```python
from build123d import *

# Parameters (mm, degrees)
SKETCH_1_W          = 71.15
SKETCH_1_H          = 94.15
EXTRUDE_1_DEPTH     = 0.55
SKETCH_2_W          = 0.55
SKETCH_2_H          = 94.15
EXTRUDE_2_DEPTH     = 9.5
SKETCH_3_W          = 10
SKETCH_3_H          = 9.6
EXTRUDE_3_DEPTH     = 0.55
SKETCH_4_R          = 1.45
CUT_EXTRUDE_1_DEPTH = 0.55
EXTRUDE_4_DEPTH     = 71.15
SKETCH_6_W          = 5.65
SKETCH_6_H          = 0.55
EXTRUDE_5_DEPTH     = 2.3


with BuildPart() as part:
    # Эскиз1 → Бобышка-Вытянуть1 (new body)
    with BuildSketch(Plane(origin=(0, 0, 0), x_dir=(1, 0, 0), z_dir=(0, 1, 0))):
        Rectangle(SKETCH_1_W, SKETCH_1_H)
    extrude(amount=EXTRUDE_1_DEPTH)

    # Эскиз2 → Бобышка-Вытянуть2 (add)
    with BuildSketch(Plane.XZ):
        with Locations((-35.3, 0)):
            Rectangle(SKETCH_2_W, SKETCH_2_H)
        with Locations((35.3, 0)):
            Rectangle(SKETCH_2_W, SKETCH_2_H)
    extrude(amount=EXTRUDE_2_DEPTH)

    # Эскиз3 → Бобышка-Вытянуть3 (add)
    with BuildSketch(Plane(origin=(0, 0.55, 0), x_dir=(1, 0, 0), z_dir=(0, 1, 0))):
        with Locations((-28.625, 51.875)):
            Rectangle(SKETCH_3_W, SKETCH_3_H)
    extrude(amount=-EXTRUDE_3_DEPTH)

    # Эскиз4 → Вырез-Вытянуть1 (cut)
    with BuildSketch(Plane(origin=(0, 0.55, 0), x_dir=(1, 0, 0), z_dir=(0, 1, 0))):
        with Locations(Location((-28.575, 51.625, 0), (0, 0, 270))):
            Circle(SKETCH_4_R)
    extrude(amount=-CUT_EXTRUDE_1_DEPTH, mode=Mode.SUBTRACT)

    # Эскиз5 → Бобышка-Вытянуть4 (add)
    with BuildSketch(Plane.ZY.offset(35.575)):
        Polygon((42.075, 0.55), (42.075, 1.1), (53.125, 1.1), (53.125, -9.5), (52.575, -9.5), (52.575, 0.55), align=None)
    extrude(amount=-EXTRUDE_4_DEPTH)

    # Эскиз6 → Бобышка-Вытянуть5 (add)
    with BuildSketch(Plane.ZY.offset(35.575)):
        with Locations((-21.9, -5.975)):
            Rectangle(SKETCH_6_W, SKETCH_6_H)
        with Locations((32.7, -5.975)):
            Rectangle(SKETCH_6_W, SKETCH_6_H)
    extrude_5 = extrude(amount=EXTRUDE_5_DEPTH)

    # Зеркальное отражение1: Бобышка-Вытянуть5 across plane
    add(extrude_5.mirror(Plane(origin=(0, 0, 0), x_dir=(0, 0, 1), z_dir=(1, 0, 0))))


solid = part.part
```
Geometry: final body of the model. Coordinates: model frame, mm. A direction names the side the tool comes from. Coordinates: 2 decimals unless noted, no trailing zeros. Order: outer loops, then holes, each group sorted by start corner. A loop starts at its lowest first (then second) coordinate and runs counter-clockwise, first axis right, second up. Notation, with made-up numbers: M -18,47.25 L -11,47.25 A20 ccw -11,79.25 Z; hole C 60.5,-13.75 d1. An arc over 180 degrees is marked long. Answer as CSV lines item,"result".
Q1. Section B-B on z = -26. Return the cut outline in (x, y) (3 decimals).
Answers:
outline,"M -35.575,-9.5 L -35.025,-9.5 L -35.025,0 L 35.025,0 L 35.025,-9.5 L 35.575,-9.5 L 35.575,0.55 L -35.575,0.55 Z"
Q2. Section D-D on x = -16. Return the cut outline in (y, z) (3 decimals).
Answers:
outline,"M -9.5,52.575 L 0.55,52.575 L 0.55,47.075 L 0,47.075 L 0,-47.075 L 0.55,-47.075 L 0.55,42.075 L 1.1,42.075 L 1.1,53.125 L -9.5,53.125 Z"
Q3. Line query: probe 1 along X at (y, z) = (-7, -0.5) (3 decimals); probe 2 along Z at (x, y) = (-21.5, 0.5) (3 decimals); probe 3 along Y at (x, z) = (18, -10.5). Output: solid intervals per line, ascending. Write a range as [from, to].
Answers:
probe 1,"x = [-35.575, -35.025], [35.025, 35.575]"
probe 2,"z = [-47.075, 47.075], [52.575, 53.125]"
probe 3,"y = [0, 0.55]"
Q4. Draft query along X for faces 1 (the flat face through (0, 0, -6)), 2 (the flat face through (-37, -5.7, 33)). Return one class per face: pulls with the +X half, pulls with the -X half, needs draft (parallel to the pull), parting line crosses it, or undercut.
Answers:
face 1,"undercut"
face 2,"needs draft"
Q5. Section C-C on x = -26. Return the cut outline in (y, z) (3 decimals), and give its area (3 significant figures).
Answers:
outline,"M -9.5,52.575 L 0.55,52.575 L 0.55,47.075 L 0,47.075 L 0,-56.675 L 0.55,-56.675 L 0.55,42.075 L 1.1,42.075 L 1.1,53.125 L -9.5,53.125 Z"
area,"68.7 mm^2"
Q6. First-contact query: P1, Ø1, axis at x = -17.5, y = -2, coming from the -Z side (3 decimals); P2, Ø3, axis at y = -5, z = 14, coming from the +X side (3 decimals); P3, Ø1.8, axis at x = 37, z = 32, coming from the -Y side; P4, Ø2.5, axis at x = -36.5, z = 32.5, coming from the -Y side. Flat tips, straight axial feed; report the tip coordinate or a pass-through.
Answers:
P1,"stops at z = 52.575"
P2,"stops at x = 35.575"
P3,"stops at y = -6.25"
P4,"stops at y = -9.5"
Q7. Set-up query: faces 3 (the flat face through (37, -5.7, 33)), 4 (the flat face through (0, 0.55, 50)), 5 (the flat face through (0, 0.55, -8)), 6 (the flat face through (35.025, -5, -1)), 7 (the flat face through (-37, -5.7, -22)). Return all of +Z, -Z, +X, -X, +Y, -Y with unobstructed straight access to the full face (end or side cutting, diameter ignored); none if empty.
Answers:
face 3,"+Z, -Z, +X, +Y"
face 4,"+X, -X, -Y"
face 5,"-Z, +X, -X, +Y"
face 6,"-Z, -Y"
face 7,"+Z, -Z, -X, +Y"
Q8. Section A-A on y = -3.75. Return the cut outline in (x, z) (3 decimals).
Answers:
outline,"M -35.575,-47.075 L -35.025,-47.075 L -35.025,47.075 L -35.575,47.075 Z; M -35.575,52.575 L 35.575,52.575 L 35.575,53.125 L -35.575,53.125 Z; M 35.025,-47.075 L 35.575,-47.075 L 35.575,47.075 L 35.025,47.075 Z"
